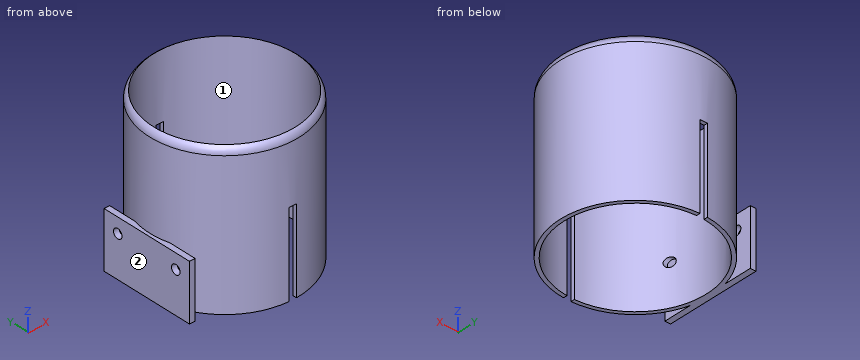
from build123d import *

# Parameters (mm, degrees)
F0_R      = 40
F1_DEPTH  = 80
F2_R      = 38
F3_DEPTH  = 90
F5_W      = 4
F5_H      = 45
F6_DEPTH  = 40
F7_W      = 3
F7_H      = 50
F8_DEPTH  = 30
F9_R      = 2.5
F10_DEPTH = 30


# Not quite as in the source:
# - a fillet or chamfer that OpenCascade refuses, or shapes differently, is made with other operations: its cross-section is extruded or revolved along the edge and cut away or added


with BuildPart() as f1:
    # F0 (on Top) → F1 (new body)
    with BuildSketch(Plane.XY):
        Circle(F0_R)
    extrude(amount=F1_DEPTH)

    # F2 (on face) → F3 (cut)
    with BuildSketch(Plane(origin=(0, 0, 0), x_dir=(1, 0, 0), z_dir=(0, 0, -1))):
        Circle(F2_R)
    extrude(amount=-F3_DEPTH, mode=Mode.SUBTRACT)

    # F4: fillet of radius 5 on 1 edges, made by hand

    # F4_s1 → F4_t2 (revolve, cut)
    with BuildSketch(Plane.XZ):
        with BuildLine():
            ThreePointArc((40, 76), (39.472135955, 78.2360679775), (38, 80))
            Line((38, 80), (40, 80))
            Line((40, 80), (40, 76))
        make_face()
    revolve(axis=Axis((0, 0, 80), (0, 0, 1)), mode=Mode.SUBTRACT)

    # F5 (on Front) → F6 (cut, symmetric)
    with BuildSketch(Plane.XZ):
        with Locations((-0.0568005547, 22.5)):
            Rectangle(F5_W, F5_H)
    extrude(amount=F6_DEPTH, both=True, mode=Mode.SUBTRACT)

    # F7 (on Top) → F8 (join)
    with BuildSketch(Plane.XY):
        with Locations((-40.154192288, 0)):
            Rectangle(F7_W, F7_H)
    extrude(amount=F8_DEPTH)

    # F9 (on face) → F10 (cut)
    with BuildSketch(Plane(origin=(-41.654192288, 0, 0), x_dir=(0, -1, 0), z_dir=(-1, 0, 0))):
        with Locations((-17, 22)):
            Circle(F9_R)
        with Locations((17, 22)):
            Circle(F9_R)
    extrude(amount=-F10_DEPTH, mode=Mode.SUBTRACT)


solid = f1.part
Could you check a few things on this model? Use its own coordinates, in mm. Face numbers are marked on the shaded views. Coordinates: 2 decimals unless noted, no trailing zeros. Order: outer loops, then holes, each group sorted by start corner. A loop starts at its lowest first (then second) coordinate and runs counter-clockwise, first axis right, second up. Notation, with made-up numbers: (63, 81) -> (75, 81) arc R18 cw to (75, 109) -> close; hole circle Ø2 at (60, 45.5). An arc over 180 degrees is marked (long way). One line per item, written item: value. Start each with the question number.
1) Imagine slicing it at A-A on y = 0. List the corners of the cut face in (x, z) for me.
2) Imagine slicing it at B-B on x = 0. List the corners of the cut face in (y, z) for me.
3) I'm going to push flat-ended pins straight in: pin 1 (1 mm diameter, centred on x = 1, y = -39.5, fed in from -Z); pin 2 (8 mm diameter, centred on y = -17, z = 22, fed in from -X); pin 3 (8 mm diameter, centred on y = 17, z = 22, fed in from +X); pin 4 (4 mm diameter, centred on x = 9.5, z = 40.5, fed in from -Y). Where does each tip first touch, or does it pass through?
4) We'd pull the mould along Y, two halves only. Please class the marked faces 1 and 2: +Y half, -Y half, draft (parallel to the pull), parting line (faces both ways), or undercut.
5) If I drill on L1, parallel to X at y = -12.5, z = 28.5; L2, parallel to X at y = -12, z = 23.5; L3, parallel to Z at x = -40, y = -17, over which ranges is the centre line in solid material (lowest first)? Write a range as [from, to].
6) Imagine slicing it at D-D on z = 53. List the corners of the cut face in (x, y) for me.
7) Imagine slicing it at C-C on z = 22. Count the separate pieces of the cut face and the enclosed holes in it, plus the area to 3 significant figures.
Answer list:
1. outline: (-41.65, 0) -> (-38, 0) -> (-38, 80) arc R5 ccw to (-40, 76) -> (-40, 30) -> (-41.65, 30) -> close; (38, 0) -> (40, 0) -> (40, 76) arc R5 ccw to (38, 80) -> close
2. outline: (-40, 45) -> (-38, 45) -> (-38, 80) arc R5 ccw to (-40, 76) -> close; (38, 45) -> (40, 45) -> (40, 76) arc R5 ccw to (38, 80) -> close
3. pin 1: stops at z = 45
3. pin 2: stops at x = -41.65
3. pin 3: stops at x = 37.83
3. pin 4: stops at y = -39.29
4. face 1: undercut
4. face 2: draft
5. L1: x = [-41.65, -38.65], [-38, -35.89], [35.89, 38]
5. L2: x = [-41.65, -38.65], [-38.16, -36.06], [36.06, 38.16]
5. L3: z = [0, 19.5], [24.5, 30]
6. outline: circle Ø80 at (0, 0); hole circle Ø76 at (0, 0)
7. separate pieces: 6
7. enclosed holes: 0
7. area: 553 mm2
